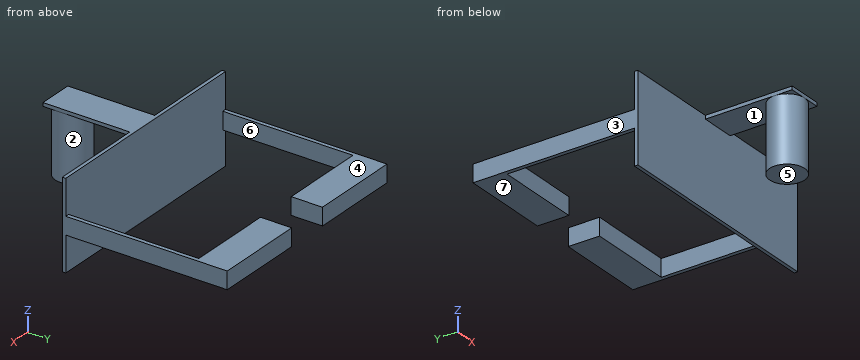
```python
from build123d import *

# Parameters (mm, degrees)
SKETCH6_W            = 10.1981
SKETCH6_H            = 1.016
BOSS_EXTRUDE3_DEPTH  = 25.4
SKETCH8_R            = 5.09905
BOSS_EXTRUDE5_DEPTH  = 19.05
SKETCH11_W           = 65.69456
SKETCH11_H           = 25.654
BOSS_EXTRUDE10_DEPTH = 1.016
SKETCH16_W           = 1.143
SKETCH16_H           = 5.08
SKETCH16_W_2         = 1.155076163
BOSS_EXTRUDE11_DEPTH = 38.0746
SKETCH17_W           = 26.52268
SKETCH17_H           = 5.08
BOSS_EXTRUDE12_DEPTH = 9.144


with BuildPart() as part:
    # Sketch6 → Boss-Extrude3 (new body)
    with BuildSketch(Plane(origin=(0, 0, 0), x_dir=(1, 0, 0), z_dir=(0, 1, 0))):
        with Locations((-12.169797761, 8.14004804)):
            Rectangle(SKETCH6_W, SKETCH6_H)
    extrude(amount=BOSS_EXTRUDE3_DEPTH)

    # Sketch8 → Boss-Extrude5 (add)
    with BuildSketch(Plane.XY.offset(-8.64804804)):
        with Locations((-12.169797761, 5.098542)):
            Circle(SKETCH8_R)
    extrude(amount=-BOSS_EXTRUDE5_DEPTH)

    # Sketch11 → Boss-Extrude10 (add)
    with BuildSketch(Plane(origin=(0, 25.4, 0), x_dir=(1, 0, 0), z_dir=(0, 1, 0))):
        with Locations((-12.150747761, 20.45904804)):
            Rectangle(SKETCH11_W, SKETCH11_H)
    extrude(amount=BOSS_EXTRUDE10_DEPTH)

    # Sketch16 → Boss-Extrude11 (add)
    with BuildSketch(Plane(origin=(0, 26.416, 0), x_dir=(1, 0, 0), z_dir=(0, 1, 0))):
        with Locations((-44.426527761, 20.45904804)):
            Rectangle(SKETCH16_W, SKETCH16_H)
        with Locations((20.118994158, 20.45904804)):
            Rectangle(SKETCH16_W_2, SKETCH16_H)
    extrude(amount=BOSS_EXTRUDE11_DEPTH)

    # Sketch17 → Boss-Extrude12 (add)
    with BuildSketch(Plane(origin=(0, 64.4906, 0), x_dir=(1, 0, 0), z_dir=(0, 1, 0))):
        with Locations((-31.736687761, 20.45904804)):
            Rectangle(SKETCH17_W, SKETCH17_H)
        with Locations((7.435192239, 20.45904804)):
            Rectangle(SKETCH17_W, SKETCH17_H)
    extrude(amount=BOSS_EXTRUDE12_DEPTH)


solid = part.part
```
CAD build for the part. Positions are in the model's coordinates, mm. Face numbers are marked on the shaded views. A direction names the side the tool comes from. Round coordinates to 2 decimals unless told otherwise and drop trailing zeros. Loops run counter-clockwise (first coordinate to the right, second up) from the corner with the lowest first, then second, coordinate; pieces in that order, holes last. Notation, with made-up numbers: (-4.5, 49) - (25.5, 49) arc R16 ccw to (25.5, 65) - close; hole circle Ø10 at (-2.75, 69.25). An arc over 180 degrees is marked (long way). Return JSON: item names as keys, results as strings. Group by question number.
Q1. Band-saw the part on D-D on z = -19.5. Give the cut face in (x, y).
Q2. Flat gauge pins, fed straight in: pin 1 Ø21 at (x, y) = (-38, 60.5) entering from +Z; pin 2 Ø3 at (x, y) = (-10.5, 14) entering from -Z; pin 3 Ø5.5 at (x, y) = (-9.5, 2.5) entering from -Z. Where does each tip first touch, or does it go through?
Q3. Two-plate mould, pull along Y, no slides. Class the marked faces 1, 2 and 3: +Y half, -Y half, draft (parallel to the pull), parting line (faces both ways), or undercut.
Q4. Drill centre lines: line 1 along Y through (x, z) = (-27, -19); line 2 along Y through (x, z) = (-10, -28); line 3 along Y through (x, z) = (-12, -24.25). Where is each one in solid material? Low to high. Write a range as [from, to].
Q5. Tool access for the marked faces 4, 5, 6 and 7: list every direction of +Z, -Z, +X, -X, +Y, -Y with a clear straight run to the whole face (end or side of a thin tool).
Q6. Band-saw the part on C-C on z = -25. Give the cut face in (x, y), plus the area to 3 significant figures.
Q7. Band-saw the part on B-B on y = 52. Give the cut face in (x, z), plus the area to 3 significant figures.
Q8. Band-saw the part on A-A on x = -29.5. Give the cut face in (y, z).
Solutions:
{
 "1": {"outline": "(-45, 25.4) - (20.7, 25.4) - (20.7, 73.63) - (-5.83, 73.63) - (-5.83, 64.49) - (19.54, 64.49) - (19.54, 26.42) - (-43.86, 26.42) - (-43.86, 64.49) - (-18.48, 64.49) - (-18.48, 73.63) - (-45, 73.63) - close; circle Ø10.2 at (-12.17, 5.1)"},
 "2": {"pin 1": "stops at z = -17.92", "pin 2": "stops at z = -8.65", "pin 3": "stops at z = -27.7"},
 "3": {"face 1": "undercut", "face 2": "undercut", "face 3": "draft"},
 "4": {"line 1": "y = [25.4, 26.42], [64.49, 73.63]", "line 2": "y = [25.4, 26.42]", "line 3": "y = [0, 10.19], [25.4, 26.42]"},
 "5": {"face 4": "+Z, +X, -X, +Y", "face 5": "-Z, +X, -X, -Y", "face 6": "+Z, -Z", "face 7": "-Z, +X, -X, +Y"},
 "6": {"outline": "(-45, 25.4) - (20.7, 25.4) - (20.7, 26.42) - (-45, 26.42) - close; circle Ø10.2 at (-12.17, 5.1)", "area": "148 mm^2"},
 "7": {"outline": "(-45, -23) - (-43.86, -23) - (-43.86, -17.92) - (-45, -17.92) - close; (19.54, -23) - (20.7, -23) - (20.7, -17.92) - (19.54, -17.92) - close", "area": "11.7 mm^2"},
 "8": {"outline": "(25.4, -33.29) - (26.42, -33.29) - (26.42, -7.63) - (25.4, -7.63) - close; (64.49, -23) - (73.63, -23) - (73.63, -17.92) - (64.49, -17.92) - close"}
}
